Can you work these out from the model? Positions are in its coordinate system, mm. Give positions to 0.01 mm unless a question says otherwise; leave off trailing zeros. Loops run counter-clockwise (first coordinate to the right, second up) from the corner with the lowest first, then second, coordinate; pieces in that order, holes last. Notation, with made-up numbers: (-39, -9) - (6, -9) arc R20 cw to (6, -1) - close; hole circle Ø11 at (10, -4.5). An arc over 180 degrees is marked (long way). Answer in a Markdown table with one row per item.
from build123d import *

# Parameters (mm, degrees)
F0_W     = 838.2
F0_H     = 203.2
F1_DEPTH = 22.225
F2_W     = 838.2
F2_H     = 9.525
F3_DEPTH = 11.1125
F5_DEPTH = 22.225


# Not quite as in the source:
# - a feature names something its author has since deleted; it is built from what else it names


with BuildPart() as f1:
    # F0 (on Top) → F1 (new body)
    with BuildSketch(Plane.XY):
        with Locations((419.1, -101.6)):
            Rectangle(F0_W, F0_H)
    extrude(amount=F1_DEPTH)

    # F2 (on face) → F3 (cut)
    with BuildSketch(Plane.XY.offset(22.225)):
        with Locations((419.1, -4.7625)):
            Rectangle(F2_W, F2_H)
    extrude(amount=-F3_DEPTH, mode=Mode.SUBTRACT)

    # F4 (on face) → F5 (cut)
    with BuildSketch(Plane.XZ.offset(203.2)):
        Polygon((438.15, 22.225), (400.05, 22.225), (405.5913148632, 0), (432.6086851368, 0), align=None)
        Polygon((45.2586851368, 0), (50.8, 22.225), (12.7, 22.225), (18.2413148632, 0), align=None)
        Polygon((825.5, 22.225), (787.4, 22.225), (792.9413148632, 0), (819.9586851368, 0), align=None)
    extrude(amount=-F5_DEPTH, mode=Mode.SUBTRACT)


solid = f1.part
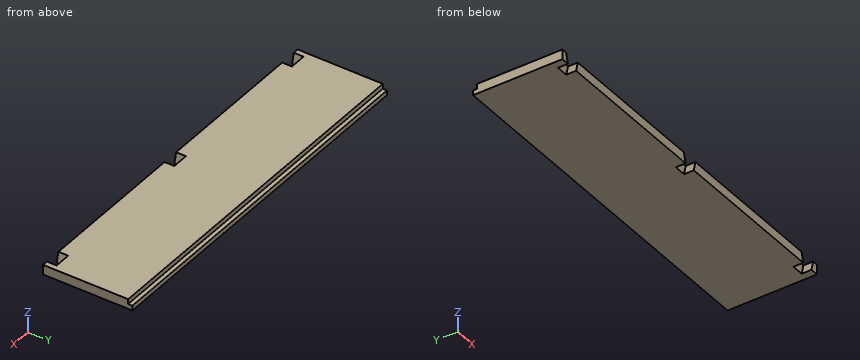
Q1. For pin 1 (6.5 mm diameter, centred on x = 38, z = 6.5, fed in from -Y) (3 decimals); pin 2 (3.5 mm diameter, centred on x = 620, z = 15, fed in from +Y) (3 decimals); pin 3 (5 mm diameter, centred on x = 226.5, y = -5, fed in from +Z), each with a flat end and sliding along its axis, tell me the tip position at first contact or that it passes through.
Checked values:
| item | result |
|---|---|
| pin 1 | stops at y = -180.975 |
| pin 2 | stops at y = -9.525 |
| pin 3 | stops at z = 11.11 |
Q2. If I drill on line 1 (Y direction, x = 675, z = 12.5) (3 decimals); line 2 (Z direction, x = 618, y = -7.5), over which ranges is the centre line in solid material (lowest first)? Write a range as [from, to].
Checked values:
| item | result |
|---|---|
| line 1 | y = [-203.2, -9.525] |
| line 2 | z = [0, 11.11] |
Q3. Imagine slicing it at B-B, the plane z = 17. Write out the boundary of the cut face in (x, y) (3 decimals).
Checked values:
| item | result |
|---|---|
| outline | (0, -203.2) - (14.003, -203.2) - (14.003, -180.975) - (49.497, -180.975) - (49.497, -203.2) - (401.353, -203.2) - (401.353, -180.975) - (436.847, -180.975) - (436.847, -203.2) - (788.703, -203.2) - (788.703, -180.975) - (824.197, -180.975) - (824.197, -203.2) - (838.2, -203.2) - (838.2, -9.525) - (0, -9.525) - close |
Q4. Imagine slicing it at A-A, the plane x = 141.5. Write out the boundary of the cut face in (y, z) (1 decimal), and give its area (3 significant figures).
Checked values:
| item | result |
|---|---|
| outline | (-203.2, 0) - (0, 0) - (0, 11.1) - (-9.5, 11.1) - (-9.5, 22.2) - (-203.2, 22.2) - close |
| area | 4,410 mm² |
